Verification items for the finished model (mm, model axes). A direction names the side the tool comes from. Round coordinates to 2 decimals unless told otherwise and drop trailing zeros. Order: outer loops, then holes, each group sorted by start corner. A loop starts at its lowest first (then second) coordinate and runs counter-clockwise, first axis right, second up. Notation, with made-up numbers: (24.25, -31.5) -> (77.25, -31.5) arc R28 ccw to (77.25, -9.5) -> close; hole circle Ø3 at (-16, 70). An arc over 180 degrees is marked (long way). Answer in a Markdown table with one row per item. Add a question column.
```python
from build123d import *

# Parameters (mm, degrees)
IZIM1_W                     = 106
IZIM1_H                     = 76
IZIM1_R                     = 3.5
Y_KSEKLIK_EKSTR_ZYON2_DEPTH = 2.5
IZIM5_W                     = 62.3
IZIM5_H                     = 48.5
KES_EKSTR_ZYON1_DEPTH       = 2.5
Y_KSEKLIK_EKSTR_ZYON6_DEPTH = 4
RADYUS7_R                   = 3
RADYUS15_R                  = 3
IZIM12_W                    = 15
IZIM12_H                    = 4.6
IZIM12_W_2                  = 5.8
IZIM12_H_2                  = 1.25
IZIM12_W_3                  = 2
IZIM12_H_3                  = 3.95
KES_EKSTR_ZYON3_DEPTH       = 4
RADYUS16_R                  = 2.3
KES_EKSTR_ZYON5_START       = -0.5
KES_EKSTR_ZYON5_DEPTH       = 0.5
RADYUS17_R                  = 1.5


with BuildPart() as part:
    # Çizim1 → Yükseklik-Ekstrüzyon2 (new body)
    with BuildSketch(Plane.XY):
        with Locations((53, 38)):
            Rectangle(IZIM1_W, IZIM1_H)
        with Locations((55, 10.31)):
            Circle(IZIM1_R, mode=Mode.SUBTRACT)
        with Locations((69, 10.31)):
            Circle(IZIM1_R, mode=Mode.SUBTRACT)
    extrude(amount=Y_KSEKLIK_EKSTR_ZYON2_DEPTH)

    # Çizim5 → Kes-Ekstrüzyon1 (cut)
    with BuildSketch(Plane.XY.offset(2.5)):
        with Locations((49.4, 47.05)):
            Rectangle(IZIM5_W, IZIM5_H)
    extrude(amount=-KES_EKSTR_ZYON1_DEPTH, mode=Mode.SUBTRACT)

    # Çizim7 → Yükseklik-Ekstrüzyon6 (add)
    with BuildSketch(Plane(origin=(0, 0, 0), x_dir=(-1, 0, 0), z_dir=(0, 0, -1))):
        Polygon((-103.5, 73.5), (-97.5, 73.5), (-97.5, 71), (-101, 71), (-101, 67.5), (-103.5, 67.5), align=None)
        Polygon((-2.5, 2.5), (-8.5, 2.5), (-8.5, 5), (-5, 5), (-5, 8.5), (-2.5, 8.5), align=None)
        Polygon((-2.5, 67.5), (-2.5, 73.5), (-8.5, 73.5), (-8.5, 71), (-5, 71), (-5, 67.5), align=None)
        Polygon((-103.5, 8.5), (-103.5, 2.5), (-97.5, 2.5), (-97.5, 5), (-101, 5), (-101, 8.5), align=None)
    extrude(amount=Y_KSEKLIK_EKSTR_ZYON6_DEPTH)

    # Radyus7
    radyus7_edges = [part.edges().sort_by_distance(p)[0] for p in [
        (2.5, 2.5, -2),
        (2.5, 73.5, -2),
        (103.5, 2.5, -2),
        (103.5, 73.5, -2),
    ]]
    fillet(radyus7_edges, radius=RADYUS7_R)

    # Radyus15
    radyus15_edges = [part.edges().sort_by_distance(p)[0] for p in [
        (0, 76, 1.25),
        (106, 76, 1.25),
        (106, 0, 1.25),
        (0, 0, 1.25),
    ]]
    fillet(radyus15_edges, radius=RADYUS15_R)

    # Çizim12 → Kes-Ekstrüzyon3 (cut)
    with BuildSketch(Plane.XY.offset(2.5)):
        with Locations((85.15, 7.39)):
            Rectangle(IZIM12_W, IZIM12_H)
        with Locations((97.3, 13.695)):
            Rectangle(IZIM12_W_2, IZIM12_H_2)
        with Locations((99.1, 63.555)):
            Rectangle(IZIM12_W_3, IZIM12_H_3)
    extrude(amount=-KES_EKSTR_ZYON3_DEPTH, mode=Mode.SUBTRACT)

    # Radyus16
    radyus16_edges = [part.edges().sort_by_distance(p)[0] for p in [
        (92.65, 5.09, 1.25),
        (92.65, 9.69, 1.25),
        (77.65, 9.69, 1.25),
        (77.65, 5.09, 1.25),
    ]]
    fillet(radyus16_edges, radius=RADYUS16_R - 0.0001)  # a hair under: the kernel refuses the full size

    # Çizim14 → Kes-Ekstrüzyon5 (cut)
    with BuildSketch(Plane(origin=(0, 0, 0), x_dir=(-1, 0, 0), z_dir=(0, 0, -1)).offset(KES_EKSTR_ZYON5_START)):
        with BuildLine():
            Line((-106, 3), (-105, 3))
            ThreePointArc((-105, 3), (-104.414213562, 1.585786438), (-103, 1))
            Line((-103, 1), (-103, 0))
            ThreePointArc((-103, 0), (-105.121320344, 0.878679656), (-106, 3))
        make_face()
        with BuildLine():
            Line((-3, 1), (-3, 0))
            ThreePointArc((-3, 0), (-0.878679656, 0.878679656), (0, 3))
            Line((0, 3), (-1, 3))
            ThreePointArc((-1, 3), (-1.585786438, 1.585786438), (-3, 1))
        make_face()
        with BuildLine():
            Line((-3, 76), (-3, 75))
            ThreePointArc((-3, 75), (-1.585786438, 74.414213562), (-1, 73))
            Line((-1, 73), (0, 73))
            ThreePointArc((0, 73), (-0.878679656, 75.121320344), (-3, 76))
        make_face()
    extrude(amount=KES_EKSTR_ZYON5_DEPTH, mode=Mode.SUBTRACT)

    # Radyus17
    radyus17_edges = [part.edges().sort_by_distance(p)[0] for p in [
        (3.75, 8.5, 0),
        (5, 6.75, 0),
        (6.75, 5, 0),
        (8.5, 3.75, 0),
        (3.75, 67.5, 0),
        (8.5, 72.25, 0),
        (6.75, 71, 0),
        (5, 69.25, 0),
        (102.25, 8.5, 0),
        (97.5, 3.75, 0),
        (99.25, 5, 0),
        (101, 6.75, 0),
        (102.25, 67.5, 0),
        (101, 69.25, 0),
        (99.25, 71, 0),
        (97.5, 72.25, 0),
    ]]
    fillet(radyus17_edges, radius=RADYUS17_R)


solid = part.part
```
1) Cross-section at A-A, the plane x = 55. Record the boundary of the cut face in (y, z).
2) Draft check along Y on faces 5 (the face through (1.6, 74.43, 0.25)), 6 (the face through (0, 38, 1)), 7 (the face through (99, 71, -3)). Enter one of: +Y half, -Y half, draft (parallel to the pull), parting line (faces both ways), or undercut.
3) Depth check by flat-ended pin: P1, Ø2, axis at x = 6, z = -2.5, coming from the -Y side; P2, Ø2.5, axis at x = 1, y = 1, coming from the -Z side; P3, Ø0.8, axis at y = 3.5, z = -3, coming from the +X side. Enter the tip coordinate at first touch or a pass-through.
4) Tool access check on faces 1 (the face through (99, 5, -3)), 2 (the face through (1.57, 1.6, 0.25)), 3 (the face through (91.99, 9, 1.23)), 4 (the face through (7, 2.5, -2)). Record the directions out of +Z, -Z, +X, -X, +Y, -Y that give a thin tool (end or side, any length) a straight path to the whole face; none if there is none.
5) Cross-section at D-D, the plane y = 17. Record the boundary of the cut face in (x, z), and give its area (3 significant figures).
6) Thickness scan on L1, parallel to Y at x = 55, z = 1.05; L2, parallel to Y at x = 22, z = 2.25; L3, parallel to Y at x = 99, z = 0.25. Record the ranges inside material, lowest first. Write a range as [from, to].
7) Cross-section at B-B, the plane y = 45. Record the boundary of the cut face in (x, z).
8) Cross-section at C-C, the plane z = -2.5. Record the boundary of the cut face in (x, y).
Results below:
| question | item | result |
|---|---|---|
| 1 | outline | (0, 0) -> (6.81, 0) -> (6.81, 2.5) -> (0, 2.5) -> close; (13.81, 0) -> (22.8, 0) -> (22.8, 2.5) -> (13.81, 2.5) -> close; (71.3, 0) -> (76, 0) -> (76, 2.5) -> (71.3, 2.5) -> close |
| 2 | face 5 | +Y half |
| 2 | face 6 | draft |
| 2 | face 7 | undercut |
| 3 | P1 | y = 2.5 |
| 3 | P2 | z = 0 |
| 3 | P3 | x = 103.04 |
| 4 | face 1 | -Z |
| 4 | face 2 | -Z, -X, -Y |
| 4 | face 3 | +Z, -Z |
| 4 | face 4 | -Z, +X, -X, -Y |
| 5 | outline | (0, 0) -> (106, 0) -> (106, 2.5) -> (0, 2.5) -> close |
| 5 | area | 265 mm² |
| 6 | L1 | [0, 6.81], [13.81, 22.8], [71.3, 76] |
| 6 | L2 | [0, 22.8], [71.3, 76] |
| 6 | L3 | [0, 13.07], [14.32, 61.58], [65.53, 76] |
| 7 | outline | (0, 0) -> (18.25, 0) -> (18.25, 2.5) -> (0, 2.5) -> close; (80.55, 0) -> (106, 0) -> (106, 2.5) -> (80.55, 2.5) -> close |
| 8 | outline | (2.5, 5.5) arc R3 ccw to (5.5, 2.5) -> (8.5, 2.5) -> (8.5, 5) -> (5, 5) -> (5, 8.5) -> (2.5, 8.5) -> close; (2.5, 67.5) -> (5, 67.5) -> (5, 71) -> (8.5, 71) -> (8.5, 73.5) -> (5.5, 73.5) arc R3 ccw to (2.5, 70.5) -> close; (97.5, 2.5) -> (100.5, 2.5) arc R3 ccw to (103.5, 5.5) -> (103.5, 8.5) -> (101, 8.5) -> (101, 5) -> (97.5, 5) -> close; (97.5, 71) -> (101, 71) -> (101, 67.5) -> (103.5, 67.5) -> (103.5, 70.5) arc R3 ccw to (100.5, 73.5) -> (97.5, 73.5) -> close |
